from build123d import *

# Parameters (mm, degrees)
F1_DEPTH = 3


with BuildPart() as f1:
    # F0 (on Front) → F1 (new body)
    with BuildSketch(Plane.XZ):
        with BuildLine():
            Line((-27.000000372, 67.3308055204), (-27.0000003572, 60.5094830675))
            add(Edge.make_bspline(
                [(-27.0000003783, 70.2132413448), (-27.000000372, 67.3308055204), (-26.8073760372, 64.0094927256), (-27.0000003572, 60.5094830675)],
                knots=[0, 0, 0, 0, 0.0797949898, 0.0797949898, 0.0797949898, 0.0797949898], degree=3))
            Line((-27.0000003783, 70.2132413448), (-27.000000372, 67.3308055204))
        make_face()
        with BuildLine():
            add(Edge.make_bspline(
                [(-27.0000003783, 70.2132413448), (-27.000000372, 67.3308055204), (-26.8073760372, 64.0094927256), (-27.0000003572, 60.5094830675)],
                knots=[0, 0, 0, 0, 0.0797949898, 0.0797949898, 0.0797949898, 0.0797949898], degree=3))
            add(Edge.make_bspline(
                [(-27.0000003572, 60.5094830675), (-27.2115741289, 56.665159338), (-28.5032848349, 48.9114242757), (-30.7959376047, 39.269131214), (-32.7990054786, 33.0934715655), (-33.9583066177, 28.9822912379)],
                knots=[0.0797949898, 0.0797949898, 0.0797949898, 0.0797949898, 0.1674398258, 0.2471817217, 0.3319487208, 0.3319487208, 0.3319487208, 0.3319487208], degree=3))
            add(Edge.make_bspline(
                [(-37.2038997366, 13.1717467116), (-36.2347795039, 17.9824819127), (-35.0866971891, 23.3074594843), (-33.9583066177, 28.9822912379)],
                knots=[0.7969356306, 0.7969356306, 0.7969356306, 0.7969356306, 1, 1, 1, 1], degree=3))
            add(Edge.make_bspline(
                [(-37.2038997366, 13.1717467116), (-37.3377860295, 11.7966552771), (-37.8318020205, 3.6131566189), (-34.8319401075, -9.4971781129), (-33.3481357614, -22.2384102756), (-27.0171200398, -42.5814503212), (-25.8644027957, -62.9931088525), (-25.7257572716, -70.2838279012)],
                knots=[0.4247645948, 0.4247645948, 0.4247645948, 0.4247645948, 0.4471809961, 0.5577287405, 0.6473745734, 0.7857235681, 0.8551599855, 0.8551599855, 0.8551599855, 0.8551599855], degree=3))
            ThreePointArc((-25.7257572716, -70.2838279012), (-24.1356221819, -86.7785971976), (-26.2738365605, -103.2113079605))
            add(Edge.make_bspline(
                [(-26.2738365605, -103.2113079605), (-26.4866600906, -108.6415730769), (-26.7346990947, -114.1409528022), (-26.9831408055, -119.6440920773)],
                knots=[0.952812329, 0.952812329, 0.952812329, 0.952812329, 0.9989562439, 0.9989562439, 0.9989562439, 0.9989562439], degree=3))
            Line((-26.9831408055, -119.6440920773), (0, -119.6440920773))
            Line((-6.3e-09, -119.6440920772), (26.9834561434, -119.6440920746))
            add(Edge.make_bspline(
                [(26.7797560592, -105.146393671), (26.7183865925, -110.0484100554), (26.7770637598, -114.8950679943), (26.9834561434, -119.6440920746)],
                knots=[0.9591803486, 0.9591803486, 0.9591803486, 0.9591803486, 0.9989568231, 0.9989568231, 0.9989568231, 0.9989568231], degree=3))
            ThreePointArc((26.7797560592, -105.146393671), (24.3110117736, -80.3279975292), (30.2677449554, -56.1088973147))
            ThreePointArc((30.2677449554, -56.1088973147), (29.3582502263, -44.7091117977), (33.0959109358, -33.901143306))
            add(Edge.make_bspline(
                [(37.3760657429, 12.312352727), (37.4207370145, 11.2848759506), (37.6386418394, 0.6550807977), (35.3777267818, -16.2805465578), (33.0959109358, -33.901143306)],
                knots=[0.5873705512, 0.5873705512, 0.5873705512, 0.5873705512, 0.6053891461, 0.7637611434, 0.7637611434, 0.7637611434, 0.7637611434], degree=3))
            add(Edge.make_bspline(
                [(37.3760657429, 12.312352727), (36.3723917785, 17.3454447873), (35.1543287191, 22.9673311954), (33.9583066177, 28.9822912379)],
                knots=[0.7847647083, 0.7847647083, 0.7847647083, 0.7847647083, 1, 1, 1, 1], degree=3))
            add(Edge.make_bspline(
                [(27.0000003572, 60.5094830675), (27.211196853, 56.9686043212), (28.5006041901, 48.7178368751), (30.8051136621, 39.5194264195), (32.7778690192, 32.6057451698), (33.9583066177, 28.9822912379)],
                knots=[0.1080256566, 0.1080256566, 0.1080256566, 0.1080256566, 0.2266783563, 0.3346321349, 0.449388848, 0.449388848, 0.449388848, 0.449388848], degree=3))
            add(Edge.make_bspline(
                [(27.0000003783, 70.2132413448), (27.0000003698, 66.3110286441), (26.8077195227, 63.7332255726), (27.0000003572, 60.5094830675)],
                knots=[0, 0, 0, 0, 0.1080256566, 0.1080256566, 0.1080256566, 0.1080256566], degree=3))
            ThreePointArc((27.0000003783, 70.2132413448), (24.5597225455, 81.642003215), (27.0140844765, 93.0677487616))
            Line((27.0140844765, 93.0677487616), (27.0165528594, 97.073236044))
            Line((27.0165528594, 97.073236044), (27.0165528594, 126.5655265976))
            ThreePointArc((27.0165528594, 126.5655265976), (26.2369988642, 128.9421564287), (24.1982364647, 130.3911290521))
            ThreePointArc((24.1982364647, 130.3911290521), (18.8821286754, 131.8789775648), (13.4760826795, 132.9967261563))
            Line((13.4760826795, 132.9967261563), (13.4760826795, 111.3308812648))
            ThreePointArc((13.4760826795, 111.3308812648), (0.4287985626, 97.7135570783), (-13.4581639711, 110.4734713575))
            ThreePointArc((-13.4581639711, 110.4734713575), (-13.4768872509, 111.1836209893), (-13.4581639711, 111.8937706212))
            Line((-13.4581639711, 111.8937706212), (-13.4581639711, 132.9915701483))
            ThreePointArc((-13.4581639711, 132.9915701483), (-18.8878136613, 131.8714457801), (-24.2268647008, 130.3780240861))
            ThreePointArc((-24.2268647008, 130.3780240861), (-26.2446496183, 128.9275955182), (-27.0165494938, 126.5655265976))
            Line((-27.0165494938, 126.5655265976), (-27.0165494938, 97.073236044))
            Line((-27.0165494938, 97.073236044), (-27.0094336483, 93.0702374443))
            ThreePointArc((-27.0094336483, 93.0702374443), (-24.5568387649, 81.642749654), (-27.0000003783, 70.2132413448))
        make_face()
        with BuildLine():
            add(Edge.make_bspline(
                [(-37.2038997366, 13.1717467116), (-37.3377860295, 11.7966552771), (-37.8318020205, 3.6131566189), (-34.8319401075, -9.4971781129), (-33.3481357614, -22.2384102756), (-27.0171200398, -42.5814503212), (-25.8644027957, -62.9931088525), (-25.7257572716, -70.2838279012)],
                knots=[0.4247645948, 0.4247645948, 0.4247645948, 0.4247645948, 0.4471809961, 0.5577287405, 0.6473745734, 0.7857235681, 0.8551599855, 0.8551599855, 0.8551599855, 0.8551599855], degree=3))
            add(Edge.make_bspline(
                [(-36.4695142582, -29.3788072578), (-37.5997978701, -23.1616359537), (-39.5544950983, -12.3662754957), (-40.0648496415, -1.9518214908), (-38.2132158377, 8.1614782915), (-37.2038997366, 13.1717467116)],
                knots=[0, 0, 0, 0, 0.3165678715, 0.5854488298, 0.7969356306, 0.7969356306, 0.7969356306, 0.7969356306], degree=3))
            ThreePointArc((-36.4695142582, -29.3788072578), (-29.8578197059, -41.9292933744), (-30.2677449554, -56.1088973147))
            ThreePointArc((-30.2677449554, -56.1088973147), (-27.6377010863, -63.081314369), (-25.7257572716, -70.2838279012))
        make_face()
        with BuildLine():
            add(Edge.make_bspline(
                [(-26.2738365605, -103.2113079605), (-26.4866600906, -108.6415730769), (-26.7346990947, -114.1409528022), (-26.9831408055, -119.6440920773)],
                knots=[0.952812329, 0.952812329, 0.952812329, 0.952812329, 0.9989562439, 0.9989562439, 0.9989562439, 0.9989562439], degree=3))
            ThreePointArc((-26.2738365605, -103.2113079605), (-28.8907910345, -111.6137859631), (-32.4913841825, -119.6440920773))
            Line((-32.4913841825, -119.6440920773), (-26.9831408055, -119.6440920773))
        make_face()
        with BuildLine():
            Line((-13.4581639711, 110.4734713575), (-13.4581639711, 111.8937706212))
            ThreePointArc((-13.4581639711, 111.8937706212), (-13.4768872509, 111.1836209893), (-13.4581639711, 110.4734713575))
        make_face()
        with BuildLine():
            add(Edge.make_bspline(
                [(26.7797560592, -105.146393671), (26.7183865925, -110.0484100554), (26.7770637598, -114.8950679943), (26.9834561434, -119.6440920746)],
                knots=[0.9591803486, 0.9591803486, 0.9591803486, 0.9591803486, 0.9989568231, 0.9989568231, 0.9989568231, 0.9989568231], degree=3))
            Line((26.9834561434, -119.6440920746), (32.4913842119, -119.644092074))
            ThreePointArc((32.4913841825, -119.6440920773), (29.2510439227, -112.5467338616), (26.7797560592, -105.146393671))
        make_face()
        with BuildLine():
            add(Edge.make_bspline(
                [(37.3760657429, 12.312352727), (37.4207370145, 11.2848759506), (37.6386418394, 0.6550807977), (35.3777267818, -16.2805465578), (33.0959109358, -33.901143306)],
                knots=[0.5873705512, 0.5873705512, 0.5873705512, 0.5873705512, 0.6053891461, 0.7637611434, 0.7637611434, 0.7637611434, 0.7637611434], degree=3))
            ThreePointArc((33.0959109358, -33.901143306), (34.6666972167, -31.5542800935), (36.4665470243, -29.37811899))
            add(Edge.make_bspline(
                [(36.4665470243, -29.37811899), (37.596826169, -23.1609722577), (39.5556506505, -12.3664838808), (40.0569196281, -2.1108359245), (38.3055086703, 7.651504698), (37.3760657429, 12.312352727)],
                knots=[0, 0, 0, 0, 0.3165666204, 0.5854480709, 0.7847647083, 0.7847647083, 0.7847647083, 0.7847647083], degree=3))
        make_face()
        with BuildLine():
            add(Edge.make_bspline(
                [(27.0000003783, 70.2132413448), (27.0000003698, 66.3110286441), (26.8077195227, 63.7332255726), (27.0000003572, 60.5094830675)],
                knots=[0, 0, 0, 0, 0.1080256566, 0.1080256566, 0.1080256566, 0.1080256566], degree=3))
            Line((27.0000003572, 60.5094830675), (27.0000003783, 70.2132413448))
        make_face()
    extrude(amount=F1_DEPTH)


solid = f1.part
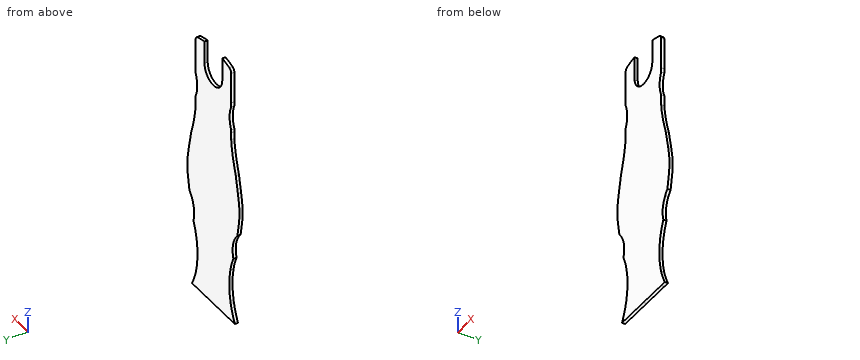
Here's how the part is built. I have some questions about the finished solid (model axes, mm). Give positions to 0.01 mm unless a question says otherwise; leave off trailing zeros. Order: outer loops, then holes, each group sorted by start corner. A loop starts at its lowest first (then second) coordinate and runs counter-clockwise, first axis right, second up. Notation, with made-up numbers: M 83.25,51 L 103.25,51 A26 ccw 103.25,84 Z; hole C 47.5,-36 d4. An arc over 180 degrees is marked long. Answer as a JSON object with one key per item and string values. Group by question number.
1) Suppose I cut it at B-B, the plane z = -88. Write out the boundary of the cut face in (x, y), plus the area to 3 significant figures.
2) I'm going to push flat-ended pins straight in: pin 1 Ø5 at (x, z) = (30.5, 71.5) entering from -Y; pin 2 Ø1.5 at (y, z) = (-2, 63) entering from -X; pin 3 Ø8 at (x, z) = (22.5, -89) entering from +Y; pin 4 Ø1.5 at (x, y) = (1.5, -2.5) entering from +Z. Where does each tip first touch, or does it pass through?
3) Please list where these lines run through material, in increasing order: L1, parallel to X at y = -1.65, z = 114; L2, parallel to X at y = -0.15, z = 109; L3, parallel to X at y = -1.25, z = -83.5. Write a range as [from, to].
4) Suppose I cut it at A-A, the plane x = -10. Write out the boundary of the cut face in (y, z), plus the area to 3 significant figures.
Results found:
{
 "1": {"outline": "M -24.17,-3 L 24.17,-3 L 24.17,0 L -24.17,0 Z", "area": "145 mm²"},
 "2": {"pin 1": "through", "pin 2": "x = -27", "pin 3": "y = 0", "pin 4": "z = 97.9"},
 "3": {"L1": "[-27.02, -13.46], [13.48, 27.02]", "L2": "[-27.02, -13.3], [13.3, 27.02]", "L3": "[-24.15, 24.15]"},
 "4": {"outline": "M -3,-119.64 L 0,-119.64 L 0,102.15 L -3,102.15 Z", "area": "665 mm²"}
}
